from build123d import *

# Parameters (mm, degrees)
SKETCH1_W                      = 266.7
SKETCH1_H                      = 228.6
BOSS_EXTRUDE1_DEPTH            = 6.35
M4_CLEARANCE_HOLE1_D           = 4.8
M4_CLEARANCE_HOLE1_DEPTH       = 6.35
M4_CLEARANCE_HOLE1_CSINK_D     = 4.85
M4_CLEARANCE_HOLE1_CSINK_ANGLE = 90


with BuildPart() as part:
    # Sketch1 → Boss-Extrude1 (new body)
    with BuildSketch(Plane(origin=(0, 0, 0), x_dir=(1, 0, 0), z_dir=(0, 1, 0))):
        Rectangle(SKETCH1_W, SKETCH1_H)
    extrude(amount=BOSS_EXTRUDE1_DEPTH)

    # M4 Clearance Hole1
    with Locations(Plane(origin=(0, 6.35, 0), x_dir=(1, 0, 0), z_dir=(0, 1, 0))):
        with Locations((123.125, 103.9), (91.125, 103.9), (91.125, 73.9), (123.125, -53.1), (123.125, -23.1), (123.125, 73.9), (-123.125, 103.9), (-91.125, 103.9), (-91.125, 73.9), (91.125, -53.1), (-123.125, -53.1), (-91.125, -53.1), (-91.125, -23.1), (-123.125, -23.1), (-123.125, 73.9), (91.125, -23.1)):
            CounterSinkHole(M4_CLEARANCE_HOLE1_D / 2, M4_CLEARANCE_HOLE1_CSINK_D / 2, depth=M4_CLEARANCE_HOLE1_DEPTH, counter_sink_angle=M4_CLEARANCE_HOLE1_CSINK_ANGLE)


solid = part.part
Could you check a few things on this model? Use its own coordinates, in mm. Round coordinates to 2 decimals unless told otherwise and drop trailing zeros. Write item = value, one per line.
1) I'm going to push a flat-ended pin straight in: P1, Ø4, axis at x = -123.125, z = -73.9, coming from the -Y side. Where does the tip first touch, or does it pass through?
Computed:
P1 = through
2) If we mould it in two halves opening along X, with no side actions, what happens to faces 1 (the flat face through (-133.35, 3, 2)), 2 (the flat face through (133.35, 3, 2)), 3 (the flat face through (-2, 3, -114.3))? For each: pulls with the +X half, pulls with the -X half, needs draft (parallel to the pull), parting line crosses it, or undercut.
Computed:
face_1 = pulls with the -X half
face_2 = pulls with the +X half
face_3 = needs draft
3) I need wall thicknesses on line 1 along X through (y, z) = (2.5, 23.1) (3 decimals); line 2 along Z through (x, y) = (-122, 1.75); line 3 along X through (y, z) = (1.25, 22). Which ranges of each line are inside material? Lowest first, please. Write a range as from..to.
Computed:
line_1 = -133.35..-125.525, -120.725..-93.525, -88.725..88.725, 93.525..120.725, 125.525..133.35
line_2 = -114.3..-106.02, -101.78..-76.02, -71.78..20.98, 25.22..50.98, 55.22..114.3
line_3 = -133.35..-125.26, -120.99..-93.26, -88.99..88.99, 93.26..120.99, 125.26..133.35
